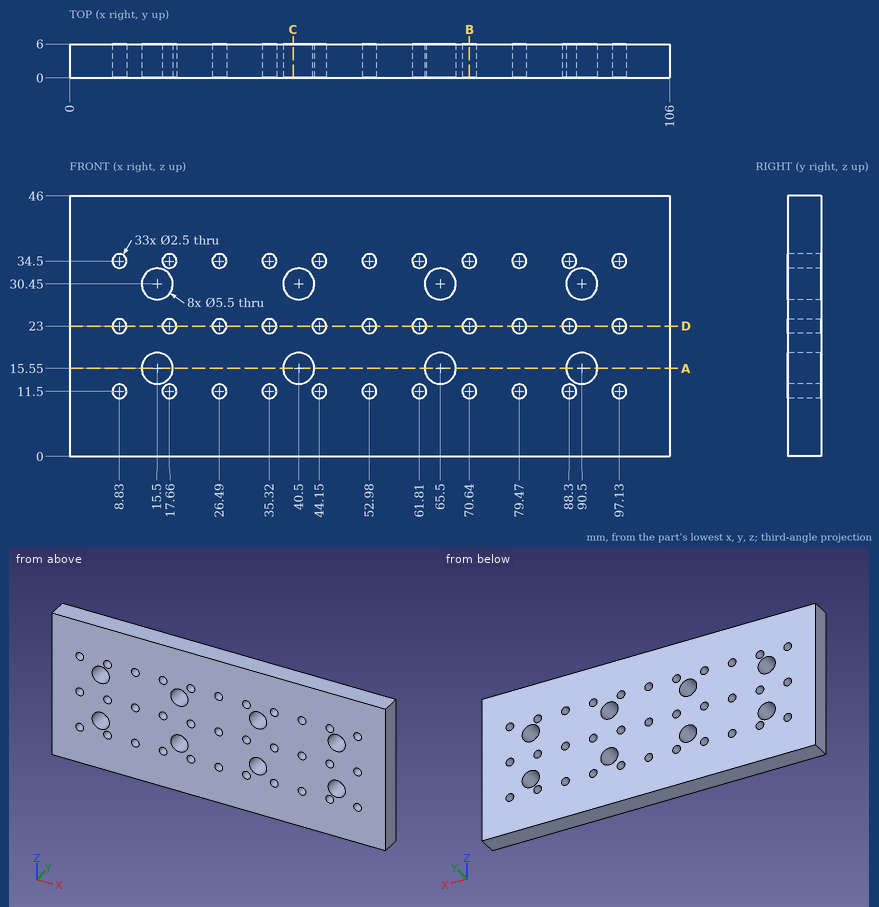
Could you check a few things on this drawing? It's one solid part, dimensions in mm from its lowest x, y, z. Give positions to 0.01 mm unless a question says otherwise; leave off trailing zeros. Order: outer loops, then holes, each group sorted by start corner. A loop starts at its lowest first (then second) coordinate and runs counter-clockwise, first axis right, second up. Notation, with made-up numbers: M 33.25,28.25 L 53.25,28.25 A33 cw 53.25,60.25 Z; hole C 12.25,-1 d4. An arc over 180 degrees is marked long. Use one line per item in the form item = value.
Item 1: If we section it at C-C, the plane x = 39.5: Write out the boundary of the cut face in (y, z), and give its area (3 significant figures).
Values follow:
outline = M 0,0 L 6,0 L 6,12.99 L 0,12.99 Z; M 0,18.11 L 6,18.11 L 6,27.89 L 0,27.89 Z; M 0,33.01 L 6,33.01 L 6,46 L 0,46 Z
area = 215 mm^2
Item 2: If I drill on line 1 along X through (y, z) = (3.8, 30.45); line 2 along Z through (x, y) = (53, 4.95); line 3 along Z through (x, y) = (52, 0.9), over which ranges is the centre line in solid material (lowest first)? Write a range as [from, to].
Values follow:
line_1 = [0, 12.75], [18.25, 37.75], [43.25, 62.75], [68.25, 87.75], [93.25, 106]
line_2 = [0, 10.25], [12.75, 21.75], [24.25, 33.25], [35.75, 46]
line_3 = [0, 10.72], [12.28, 22.22], [23.78, 33.72], [35.28, 46]
Item 3: If we section it at A-A, the plane z = 15.55: Write out the boundary of the cut face in (x, y).
Values follow:
outline = M 0,0 L 12.75,0 L 12.75,6 L 0,6 Z; M 18.25,0 L 37.75,0 L 37.75,6 L 18.25,6 Z; M 43.25,0 L 62.75,0 L 62.75,6 L 43.25,6 Z; M 68.25,0 L 87.75,0 L 87.75,6 L 68.25,6 Z; M 93.25,0 L 106,0 L 106,6 L 93.25,6 Z
Item 4: If we section it at B-B, the plane x = 70.64: Write out the boundary of the cut face in (y, z).
Values follow:
outline = M 0,0 L 6,0 L 6,10.25 L 0,10.25 Z; M 0,12.75 L 6,12.75 L 6,21.75 L 0,21.75 Z; M 0,24.25 L 6,24.25 L 6,33.25 L 0,33.25 Z; M 0,35.75 L 6,35.75 L 6,46 L 0,46 Z
Item 5: If we section it at D-D, the plane z = 23: Count the separate pieces of the cut face and the enclosed holes in it, and give its area (3 significant figures).
Values follow:
separate_pieces = 12
enclosed_holes = 0
area = 471 mm^2
